from build123d import *

# Parameters (mm, degrees)
SKETCH1_W                      = 31.75
SKETCH1_H                      = 31.75
BOSS_EXTRUDE1_DEPTH            = 7.9375
CBORE_FOR_M2_SHCS1_D           = 2.4
CBORE_FOR_M2_SHCS1_CBORE_D     = 4.4
CBORE_FOR_M2_SHCS1_CBORE_DEPTH = 2


with BuildPart() as part:
    # Sketch1 → Boss-Extrude1 (new body, symmetric)
    with BuildSketch(Plane.XY):
        Rectangle(SKETCH1_W, SKETCH1_H)
    extrude(amount=BOSS_EXTRUDE1_DEPTH, both=True)

    # CBORE for M2 SHCS1 (through all)
    with Locations(Plane.XY.offset(7.9375)):
        with Locations((-11.875, 11.875), (11.875, 11.875), (11.875, -11.875), (-11.875, -11.875)):
            CounterBoreHole(CBORE_FOR_M2_SHCS1_D / 2, CBORE_FOR_M2_SHCS1_CBORE_D / 2, CBORE_FOR_M2_SHCS1_CBORE_DEPTH)


solid = part.part
Could you check a few things on this model? Use its own coordinates, in mm. A direction names the side the tool comes from. Round coordinates to 2 decimals unless told otherwise and drop trailing zeros. Order: outer loops, then holes, each group sorted by start corner. A loop starts at its lowest first (then second) coordinate and runs counter-clockwise, first axis right, second up. Notation, with made-up numbers: M 29,34 L 71,34 A28 cw 71,73 Z; hole C 7.25,80 d4. An arc over 180 degrees is marked long. One line per item, written item: value.
(1) I need wall thicknesses on line 1 along X through (y, z) = (-12, -3) (3 decimals); line 2 along Y through (x, z) = (11.5, -4.5) (3 decimals); line 3 along X through (y, z) = (-12.5, 1) (3 decimals). Which ranges of each line are inside material? Lowest first, please. Write a range as from..to.
Ans:
line 1: x = -15.875..-13.068, -10.682..10.682, 13.068..15.875
line 2: y = -15.875..-13.015, -10.735..10.735, 13.015..15.875
line 3: x = -15.875..-12.899, -10.851..10.851, 12.899..15.875
(2) Which directions (+Z, -Z, +X, -X, +Y, -Y) give clear straight access to the entire face, cutting with the end or side of a thin tool? Please do faces 1 (the flat face through (13, -13, 5.938)), 2 (the cylindrical face through (11.32, -12.94, -1.1)).
Ans:
face 1: +Z
face 2: +Z, -Z
(3) I'm going to push a flat-ended pin straight in: P1, Ø3, axis at x = 11.875, y = 11.875, coming from the +Z side. Where does the tip first touch, or does it pass through?
Ans:
P1: stops at z = 5.94
(4) Imagine slicing it at B-B (z = -6.25). Write out the boundary of the cut face in (x, y) (3 decimals).
Ans:
outline: M -15.875,-15.875 L 15.875,-15.875 L 15.875,15.875 L -15.875,15.875 Z; hole C -11.875,-11.875 d2.4; hole C -11.875,11.875 d2.4; hole C 11.875,-11.875 d2.4; hole C 11.875,11.875 d2.4
(5) If we mould it in two halves opening along Y, with no side actions, what happens to faces 3 (the flat face through (0, 0, -7.938)), 4 (the flat face through (0, -15.875, 0)), 5 (the cylindrical face through (11.32, 10.81, -1.1))? For each: released by +Y, released by -Y, zero draft, split by the parting line, or undercut.
Ans:
face 3: zero draft
face 4: released by -Y
face 5: undercut
(6) Imagine slicing it at A-A (x = -12). Write out the boundary of the cut face in (y, z) (1 decimal), and give its area (3 significant figures).
Ans:
outline: M -15.9,-7.9 L -13.1,-7.9 L -13.1,5.9 L -14.1,5.9 L -14.1,7.9 L -15.9,7.9 Z; M -10.7,-7.9 L 10.7,-7.9 L 10.7,5.9 L 9.7,5.9 L 9.7,7.9 L -9.7,7.9 L -9.7,5.9 L -10.7,5.9 Z; M 13.1,-7.9 L 15.9,-7.9 L 15.9,7.9 L 14.1,7.9 L 14.1,5.9 L 13.1,5.9 Z
area: 420 mm^2
